```python
from build123d import *

# Parameters (mm, degrees)
SKETCH1_W           = 40
SKETCH1_H           = 40
BOSS_EXTRUDE1_DEPTH = 10
FILLET1_R           = 5
SKETCH2_R           = 18.5
CUT_EXTRUDE1_DEPTH  = 11
SKETCH3_R           = 1.5
CUT_EXTRUDE2_DEPTH  = 11


with BuildPart() as part:
    # Sketch1 → Boss-Extrude1 (new body)
    with BuildSketch(Plane(origin=(0, 0, 0), x_dir=(1, 0, 0), z_dir=(0, 1, 0))):
        Rectangle(SKETCH1_W, SKETCH1_H)
    extrude(amount=BOSS_EXTRUDE1_DEPTH)

    # Fillet1
    fillet1_edges = [part.edges().sort_by_distance(p)[0] for p in [
        (20, 5, 20),
        (-20, 5, 20),
        (-20, 5, -20),
        (20, 5, -20),
    ]]
    fillet(fillet1_edges, radius=FILLET1_R)

    # Sketch2 → Cut-Extrude1 (cut, through all)
    with BuildSketch(Plane(origin=(0, 10, 0), x_dir=(1, 0, 0), z_dir=(0, 1, 0))):
        Circle(SKETCH2_R)
    extrude(amount=-CUT_EXTRUDE1_DEPTH, mode=Mode.SUBTRACT)

    # Sketch3 → Cut-Extrude2 (cut, through all)
    with BuildSketch(Plane(origin=(0, 10, 0), x_dir=(1, 0, 0), z_dir=(0, 1, 0))):
        with Locations((-16.5, 16.5)):
            Circle(SKETCH3_R)
        with Locations((16.5, 16.5)):
            Circle(SKETCH3_R)
        with Locations((16.5, -16.5)):
            Circle(SKETCH3_R)
        with Locations((-16.5, -16.5)):
            Circle(SKETCH3_R)
    extrude(amount=-CUT_EXTRUDE2_DEPTH, mode=Mode.SUBTRACT)


solid = part.part
```
For this review, take the finished solid that the model builds, in its own axes (mm). Round coordinates to 2 decimals unless told otherwise and drop trailing zeros. Loops run counter-clockwise (first coordinate to the right, second up) from the corner with the lowest first, then second, coordinate; pieces in that order, holes last.
Q1. Add section A-A on z = 0. Write out the cut boundary in (x, y), plus the area to 3 significant figures.
Result sheet:
outline: (-20, 0) - (-18.5, 0) - (-18.5, 10) - (-20, 10) - close; (18.5, 0) - (20, 0) - (20, 10) - (18.5, 10) - close
area: 30.0 mm2
Q2. Add section D-D on z = 16.5. Write out the cut boundary in (x, y), plus the area to 3 significant figures.
Result sheet:
outline: (-19.77, 0) - (-18, 0) - (-18, 10) - (-19.77, 10) - close; (-15, 0) - (-8.37, 0) - (-8.37, 10) - (-15, 10) - close; (8.37, 0) - (15, 0) - (15, 10) - (8.37, 10) - close; (18, 0) - (19.77, 0) - (19.77, 10) - (18, 10) - close
area: 168 mm2
Q3. Add section B-B on x = 0. Write out the cut boundary in (y, z).
Result sheet:
outline: (0, -20) - (10, -20) - (10, -18.5) - (0, -18.5) - close; (0, 18.5) - (10, 18.5) - (10, 20) - (0, 20) - close
Q4. Insertion check: pin 1 Ø2.5 at (x, z) = (-16.5, 16.5) entering from -Y. The pin has a flat end and moves straight along its axis. Give the tip position at first contact, or say it passes through.
Result sheet:
pin 1: passes through
Q5. To check wall thickness, follow line 1 along Z through (x, y) = (0, 8); line 2 along Z through (x, y) = (-16.5, 5.5). State the ranges of each line that lie inside material, in increasing order.
Result sheet:
line 1: z = -20 to -18.5, 18.5 to 20
line 2: z = -19.77 to -18, -15 to -8.37, 8.37 to 15, 18 to 19.77
Q6. Add section C-C on y = 7.75. Write out the cut boundary in (x, z).
Result sheet:
outline: (-20, -15) arc R5 ccw to (-15, -20) - (15, -20) arc R5 ccw to (20, -15) - (20, 15) arc R5 ccw to (15, 20) - (-15, 20) arc R5 ccw to (-20, 15) - close; hole circle Ø37 at (0, 0); hole circle Ø3 at (-16.5, -16.5); hole circle Ø3 at (-16.5, 16.5); hole circle Ø3 at (16.5, -16.5); hole circle Ø3 at (16.5, 16.5)
Q7. Mouldability with a two-part tool opening along X and no side actions: class faces 1 (the face through (-13.4, 0, 13.2)), 2 (the face through (-20, 5, 0)), 3 (the face through (-18, 5.07, -16.57)) as +X half, -X half, draft (parallel to the pull), parting line (faces both ways), or undercut.
Result sheet:
face 1: draft
face 2: -X half
face 3: undercut
